Source: CAD feature listing. Evaluate the final solid. Frame: model axes, mm. Give positions to 0.01 mm unless a question says otherwise; leave off trailing zeros. Order: outer loops, then holes, each group sorted by start corner. A loop starts at its lowest first (then second) coordinate and runs counter-clockwise, first axis right, second up.
1) Section A-A, the plane x = -27.75. Return loops of the section in (y, z).
2) Draft query along X for faces 1 (the face through (-49.234, 32, 7)), 2 (the face through (-23.57, 47.13, 19.93)), 3 (the face through (-30.225, 14.149, 7.395)). Return one class per face: released by +X, released by -X, zero draft, split by the parting line, or undercut.
3) Section C-C, the plane x = -32. Return loops of the section in (y, z).
4) Section B-B, the plane z = 13.75. Return loops of the section in (x, y), plus the area to 3 significant figures.
5) Material intervals for line 1 (Y direction, x = -28, z = 10.5); line 2 (Y direction, x = -27.25, z = 4.5); line 3 (Z direction, x = -22.75, y = 12), sorted ascending.
6) Section D-D, the plane y = 30.5. Return loops of the section in (x, z), plus the area to 3 significant figures.
7) First-contact query: P1, Ø2, axis at x = -25, z = 17, coming from the +Y side; P2, Ø3, axis at x = -23, z = 22, coming from the -Y side (3 decimals); P3, Ø2, axis at x = -28.58, y = 2.76, coming from the -Z side; P4, Ø6, axis at x = -38.5, z = 21.5, coming from the -Y side. Flat tips, straight axial feed; report the tip coordinate or a pass-through.
```python
from build123d import *

# Parameters (mm, degrees)
F0_R     = 1.65
F0_R_2   = 5.5
F0_R_3   = 11.1803398875
F1_DEPTH = 15
F0_R_4   = 7.6
F2_DEPTH = 25


# Not quite as in the source:
# - a feature names something its author has since deleted; it is built from what else it names


with BuildPart() as f1:
    # F0 (on Top) → F1 (new body)
    with BuildSketch(Plane.XY):
        with BuildLine():
            Line((-19.2339122487, 8.4197289313), (-19.2339122487, 53.7750689313))
            Line((-19.2339122487, 53.7750689313), (-19.2339122487, 55.4197289313))
            Line((-19.2339122487, 55.4197289313), (-49.2339122487, 55.4197289313))
            Line((-49.2339122487, 55.4197289313), (-49.2339122487, 8.4197289313))
            ThreePointArc((-49.2339122487, 8.4197289313), (-34.2339122487, -6.5802710687), (-19.2339122487, 8.4197289313))
        make_face()
        with Locations((-40.8839122487, 2.7628746818)):
            Circle(F0_R, mode=Mode.SUBTRACT)
        with Locations((-39.8907664982, 14.0765831808)):
            Circle(F0_R, mode=Mode.SUBTRACT)
        with Locations((-34.2339122487, 8.4197289313)):
            Circle(F0_R_2, mode=Mode.SUBTRACT)
        with Locations((-28.5770579992, 2.7628746818)):
            Circle(F0_R, mode=Mode.SUBTRACT)
        with Locations((-28.5770579992, 14.0765831808)):
            Circle(F0_R, mode=Mode.SUBTRACT)
        with Locations((-34.2339122487, 43.7750689313)):
            Circle(F0_R_3, mode=Mode.SUBTRACT)
    extrude(amount=F1_DEPTH)

    # F0 (on Top) → F2 (join)
    with BuildSketch(Plane.XY):
        with Locations((-34.2339122487, 43.7750689313)):
            Circle(F0_R_3)
        with Locations((-34.2339122487, 43.7750689313)):
            Circle(F0_R_4, mode=Mode.SUBTRACT)
    extrude(amount=F2_DEPTH)


solid = f1.part
```
From the geometry:
1. outline: (-5.11, 0) - (1.34, 0) - (1.34, 15) - (-5.11, 15) - close; (4.19, 0) - (12.65, 0) - (12.65, 15) - (4.19, 15) - close; (15.5, 0) - (39.81, 0) - (39.81, 25) - (34.67, 25) - (34.67, 15) - (15.5, 15) - close; (47.74, 0) - (55.42, 0) - (55.42, 15) - (52.88, 15) - (52.88, 25) - (47.74, 25) - close
2. face 1: released by -X
2. face 2: split by the parting line
2. face 3: undercut
3. outline: (-6.41, 0) - (3.39, 0) - (3.39, 15) - (-6.41, 15) - close; (13.45, 0) - (36.51, 0) - (36.51, 25) - (32.82, 25) - (32.82, 15) - (13.45, 15) - close; (51.04, 0) - (55.42, 0) - (55.42, 15) - (54.73, 15) - (54.73, 25) - (51.04, 25) - close
4. outline: (-49.23, 8.42) arc R15 ccw to (-19.23, 8.42) - (-19.23, 55.42) - (-49.23, 55.42) - close; hole circle Ø3.3 at (-40.88, 2.76); hole circle Ø15.2 at (-34.23, 43.78); hole circle Ø3.3 at (-39.89, 14.08); hole circle Ø11 at (-34.23, 8.42); hole circle Ø3.3 at (-28.58, 2.76); hole circle Ø3.3 at (-28.58, 14.08)
4. area: 1,450 mm2
5. line 1: y = -5.22 to 1.22, 4.31 to 12.53, 15.62 to 39.43, 48.12 to 55.42
5. line 2: y = -4.86 to 1.78, 3.74 to 13.1, 15.06 to 40.78, 46.77 to 55.42
5. line 3: z = 0 to 15
6. outline: (-49.23, 0) - (-19.23, 0) - (-19.23, 15) - (-49.23, 15) - close
6. area: 450 mm2
7. P1: stops at y = 51.34
7. P2: stops at y = 38.275
7. P3: passes through
7. P4: stops at y = 32.67
